The listing builds one solid part. Answer for the finished solid, in the listing's coordinates (mm). Round coordinates to 2 decimals unless told otherwise and drop trailing zeros. Order: outer loops, then holes, each group sorted by start corner. A loop starts at its lowest first (then second) coordinate and runs counter-clockwise, first axis right, second up. Notation, with made-up numbers: M 18,74.5 L 67,74.5 A13 cw 67,84.5 Z; hole C 88.5,77 d6. An arc over 180 degrees is marked long. Write item = value, one per line. Start each with the question number.
(1) A cutting plane is placed at A-A, the plane x = 0. Determine the outline of the cut face in (y, z), and give its area (3 significant figures).
(2) A cutting plane is placed at B-B, the plane z = 1.1. Determine the outline of the cut face in (x, y).
(3) A cutting plane is placed at D-D, the plane y = -55.5. Determine the outline of the cut face in (x, z).
(4) For a pull along Y with two mould halves and no side action, classify faces 1 (the face through (-5.5, -24.9, 1)), 2 (the face through (-1, -36, 0)) as released by +Y, released by -Y, zero draft, split by the parting line, or undercut.
(5) A cutting plane is placed at C-C, the plane y = -13.5. Determine the outline of the cut face in (x, z), and give its area (3 significant figures).
(6) Each of these flat-tipped pins is pushed along its axis until it touches: pin 1 (1 mm diameter, centred on y = -54, z = 1, fed in from +X); pin 2 (0.6 mm diameter, centred on y = -66, z = 1, fed in from -X). Where does it stop, or does it pass through?
(7) Straight lines are drawn through the part: probe 1 along Y at (x, z) = (0, 0.85); probe 2 along X at (y, z) = (-5, 1.55) (3 decimals); probe 3 along Y at (x, z) = (-12, 0.6). For each, find the intervals that lie inside material, in ascending order. Write a range as from..to.
from build123d import *

# Parameters (mm, degrees)
SKETCH_1_R      = 25.5
EXTRUDE_1_DEPTH = 2


with BuildPart() as part:
    # 草图1 → 凸台-拉伸1 (new body)
    # profile 1 of 5: a face of its own
    with BuildSketch(Plane.XY):
        with BuildLine():
            Line((-30, -30), (-30, -87.891535797))
            Line((-30, -87.891535797), (30, -87.891535797))
            Line((30, -87.891535797), (30, -30))
            ThreePointArc((30, -30), (0, -42.426406871), (-30, -30))
        make_face()
    # profile 2 of 5: a face of its own
    with BuildSketch(Plane.XY):
        with BuildLine():
            Line((-30, 30), (-30, -30))
            ThreePointArc((-30, -30), (0, -42.426406871), (30, -30))
            Line((30, -30), (30, 30))
            Line((30, 30), (-30, 30))
        make_face()
        Circle(SKETCH_1_R, mode=Mode.SUBTRACT)
    # profile 3 of 5: a face of its own
    with BuildSketch(Plane.XY):
        with BuildLine():
            ThreePointArc((-30, 30), (-42.426406871, 0), (-30, -30))
            Line((-30, -30), (-30, 30))
        make_face()
    # profile 4 of 5: a face of its own
    with BuildSketch(Plane.XY):
        with BuildLine():
            Line((30, 30), (30, -30))
            ThreePointArc((30, -30), (39.196888946, -16.235883004), (42.426406871, 0))
            ThreePointArc((42.426406871, 0), (39.196888946, 16.235883004), (30, 30))
        make_face()
    # profile 5 of 5: a face of its own
    with BuildSketch(Plane.XY):
        with BuildLine():
            ThreePointArc((30, 30), (0, 42.426406871), (-30, 30))
            Line((-30, 30), (30, 30))
        make_face()
    extrude(amount=EXTRUDE_1_DEPTH)


solid = part.part
Reported:
q1.outline = M -87.89,0 L -25.5,0 L -25.5,2 L -87.89,2 Z; M 25.5,0 L 42.43,0 L 42.43,2 L 25.5,2 Z
q1.area = 159 mm²
q2.outline = M -30,-87.89 L 30,-87.89 L 30,-30 A42.43 ccw long -30,-30 Z; hole C 0,0 d51
q3.outline = M -30,0 L 30,0 L 30,2 L -30,2 Z
q4.face_1 = undercut
q4.face_2 = zero draft
q5.outline = M -40.22,0 L -21.63,0 L -21.63,2 L -40.22,2 Z; M 21.63,0 L 40.22,0 L 40.22,2 L 21.63,2 Z
q5.area = 74.4 mm²
q6.pin_1 = 30
q6.pin_2 = -30
q7.probe_1 = -87.89..-25.5, 25.5..42.43
q7.probe_2 = -42.131..-25.005, 25.005..42.131
q7.probe_3 = -87.89..-22.5, 22.5..40.69
